from build123d import *

# Parameters (mm, degrees)
FILLET1_R               = 1
CHAMFER1_SIZE           = 1
CUT_EXTRUDE1_DEPTH      = 47.610903231
CUT_EXTRUDE1_DEPTH_BACK = 47.610903231


with BuildPart() as part:
    # Sketch1 → Revolve3 (revolve)
    with BuildSketch(Plane(origin=(0, 0, 0), x_dir=(0, 0, -1), z_dir=(1, 0, 0))):
        Polygon((0, 0), (0, 17.78), (-8, 17.78), (-8, 24.13), (-15.875, 24.13), (-15.875, 0), align=None)
        Polygon((8, 17.78), (0, 17.78), (0, 0), (15.875, 0), (15.875, 24.13), (8, 24.13), align=None)
    revolve(axis=Axis((0, 0, -15.875), (0, 0, 1)))

    # Fillet1
    fillet1_edges = [part.edges().sort_by_distance(p)[0] for p in [
        (0, -24.13, -15.875),
        (0, -24.13, 15.875),
    ]]
    fillet(fillet1_edges, radius=FILLET1_R)

    # Chamfer1
    chamfer1_edges = [part.edges().sort_by_distance(p)[0] for p in [
        (0, -24.13, -8),
        (0, -24.13, 8),
    ]]
    chamfer(chamfer1_edges, length=CHAMFER1_SIZE)

    # Sketch2 → Cut-Extrude1 (cut, two sides: drawn at the far end of the back side and taken through both)
    with BuildSketch(Plane.XY.offset(15.875).offset(-CUT_EXTRUDE1_DEPTH_BACK)):
        Polygon((7.332348419, 0), (3.666174209, 6.35), (-3.666174209, 6.35), (-7.332348419, 0), (-3.666174209, -6.35), (3.666174209, -6.35), align=None)
    extrude(amount=CUT_EXTRUDE1_DEPTH + CUT_EXTRUDE1_DEPTH_BACK, mode=Mode.SUBTRACT)


solid = part.part
Model file for the job. Use its own axes, mm. A direction names the side the tool comes from. Round coordinates to 2 decimals unless told otherwise and drop trailing zeros. Loops run counter-clockwise (first coordinate to the right, second up) from the corner with the lowest first, then second, coordinate; pieces in that order, holes last. Notation, with made-up numbers: (26.25, 14.25) -> (65.25, 14.25) arc R21 cw to (65.25, 18.25) -> close; hole circle Ø7 at (62, 3.25). An arc over 180 degrees is marked (long way). Answer as CSV lines item,"result". Start each with the question number.
1) Slice it at A-A (x = 0). List the corners of the cut face in (y, z) (3 decimals), plus the area to 3 significant figures.
2) Pin check, flat tips, straight feed: P1, Ø6, axis at y = 12.5, z = 4, coming from the +X side; P2, Ø6, axis at y = -13.5, z = -1, coming from the -X side; P3, Ø4, axis at x = -15.5, z = 10.5, coming from the -Y side. Stop position of each tip, or through.
3) Tool access for faces 1 (the face through (17, 7, -8)), 2 (the face through (5, 5, 15.875)), 3 (the face through (0, -6.35, 0)): list every direction of +Z, -Z, +X, -X, +Y, -Y with a clear straight run to the whole face (end or side of a thin tool).
4) Probe line 1 along Z through (x, y) = (19, -6) (3 decimals); line 2 along Y through (x, z) = (0, -7.5); line 3 along Z through (x, y) = (-7.5, 22.5). List the from-to ranges inside material, lowest first.
5) Slice it at B-B (z = -0.5). List the corners of the cut face in (x, y), plus the area to 3 significant figures.
6) Mould opens along X. For faces 4 (the face through (-7.248, 23.016, -11.896)), 5 (the face through (0, 6.35, 0)), 6 (the face through (5, -5, -15.875)), 7 (the face through (5.525, 3.131, -0.222)) say: +X half, -X half, draft (parallel to the pull), parting line (faces both ways), or undercut.
Filled in:
1,outline,"(-24.13, -14.875) arc R1 ccw to (-23.13, -15.875) -> (-6.35, -15.875) -> (-6.35, 15.875) -> (-23.13, 15.875) arc R1 ccw to (-24.13, 14.875) -> (-24.13, 9) -> (-23.13, 8) -> (-17.78, 8) -> (-17.78, -8) -> (-23.13, -8) -> (-24.13, -9) -> close; (6.35, -15.875) -> (23.13, -15.875) arc R1 ccw to (24.13, -14.875) -> (24.13, -9) -> (23.13, -8) -> (17.78, -8) -> (17.78, 8) -> (23.13, 8) -> (24.13, 9) -> (24.13, 14.875) arc R1 ccw to (23.13, 15.875) -> (6.35, 15.875) -> close"
1,area,"923 mm2"
2,P1,"stops at x = 15.03"
2,P2,"stops at x = -14.35"
2,P3,"stops at y = -20"
3,face 1,"none"
3,face 2,"+Z, +X, -X, +Y, -Y"
3,face 3,"+Z, -Z"
4,line 1,"z = -15.875 to -8, 8 to 15.875"
4,line 2,"y = -17.78 to -6.35, 6.35 to 17.78"
4,line 3,"z = -15.68 to -8.59, 8.59 to 15.68"
5,outline,"circle Ø35.56 at (0, 0); hole (-7.33, 0) -> (-3.67, -6.35) -> (3.67, -6.35) -> (7.33, 0) -> (3.67, 6.35) -> (-3.67, 6.35) -> close"
5,area,"853 mm2"
6,face 4,"parting line"
6,face 5,"undercut"
6,face 6,"draft"
6,face 7,"undercut"
